```python
from build123d import *

# Parameters (mm, degrees)
F0_W     = 190
F0_H     = 10
F1_DEPTH = 20
F2_R     = 3
F2_W     = 150
F2_H     = 2
F3_DEPTH = 10
F4_R     = 2.5
F5_DEPTH = 10
F6_R     = 2.5
F7_DEPTH = 10


with BuildPart() as f1:
    # F0 (on Front) → F1 (new body)
    with BuildSketch(Plane.XZ):
        Rectangle(F0_W, F0_H)
    extrude(amount=F1_DEPTH)

    # F2 (on face) → F3 (cut)
    with BuildSketch(Plane.XY.offset(5)):
        with Locations((-56, -10)):
            Circle(F2_R)
        with Locations((-23.5, -10)):
            Circle(F2_R)
        with Locations((11.5, -10)):
            Circle(F2_R)
        with Locations((46, -10)):
            Circle(F2_R)
        with Locations((0, -19)):
            Rectangle(F2_W, F2_H)
    extrude(amount=-F3_DEPTH, mode=Mode.SUBTRACT)

    # F4 (on face) → F5 (cut)
    with BuildSketch(Plane(origin=(-95, 0, 0), x_dir=(0, -1, 0), z_dir=(-1, 0, 0))):
        with Locations((5, 0)):
            Circle(F4_R)
        with Locations((15, 0)):
            Circle(F4_R)
    extrude(amount=-F5_DEPTH, mode=Mode.SUBTRACT)

    # F6 (on face) → F7 (cut)
    with BuildSketch(Plane.YZ.offset(95)):
        with Locations((-5, 0)):
            Circle(F6_R)
        with Locations((-15, 0)):
            Circle(F6_R)
    extrude(amount=-F7_DEPTH, mode=Mode.SUBTRACT)


solid = f1.part
```
Check sheet for the modelled part. Datum: model origin and axes. Units: mm. A direction names the side the tool comes from. Round coordinates to 2 decimals unless told otherwise and drop trailing zeros. Order: outer loops, then holes, each group sorted by start corner. A loop starts at its lowest first (then second) coordinate and runs counter-clockwise, first axis right, second up. Notation, with made-up numbers: (30, 78) - (79, 78) arc R25 cw to (79, 92) - close; hole circle Ø1 at (-27, 21). An arc over 180 degrees is marked (long way). Answer as CSV lines item,"result". Start each with the question number.
1) Depth check by flat-ended pin: pin 1 (1.5 mm diameter, centred on y = -6, z = 0, fed in from +X); pin 2 (4 mm diameter, centred on x = 38.5, z = 2, fed in from -Y); pin 3 (1.5 mm diameter, centred on y = -5, z = 0.5, fed in from -X). Enter the tip coordinate at first touch or a pass-through.
2) Draft check along X on faces 1 (the face through (-1, 0, 0)), 2 (the face through (85, -5, 0)), 3 (the face through (-59, -10, 0)). Enter one of: +X half, -X half, draft (parallel to the pull), parting line (faces both ways), or undercut.
3) Scan lines: probe 1 along Y at (x, z) = (11.5, 2.5); probe 2 along X at (y, z) = (-11, 1.5); probe 3 along Z at (x, y) = (92.25, -15). Record each from-to range of solid material in increasing order.
4) Section check B-B (y = -5). Record the cut outline in (x, z).
5) Section check A-A (x = -23.5). Record the cut outline in (y, z), then the cut area to 3 significant figures.
6) Tool access check on faces 4 (the face through (90.1, -17.5, 0.1)), 5 (the face through (-1, -18, 0)), 6 (the face through (-90.1, -12.5, 0.1)), 7 (the face through (-85, -20, 0)). Record the directions out of +Z, -Z, +X, -X, +Y, -Y that give a thin tool (end or side, any length) a straight path to the whole face; none if there is none.
Determined:
1,pin 1,"x = 85"
1,pin 2,"y = -18"
1,pin 3,"x = -85"
2,face 1,"draft"
2,face 2,"+X half"
2,face 3,"undercut"
3,probe 1,"-18 to -13, -7 to 0"
3,probe 2,"-95 to -58.83, -53.17 to -26.33, -20.67 to 8.67, 14.33 to 43.17, 48.83 to 95"
3,probe 3,"-5 to -2.5, 2.5 to 5"
4,outline,"(-95, -5) - (95, -5) - (95, -2.5) - (85, -2.5) - (85, 2.5) - (95, 2.5) - (95, 5) - (-95, 5) - (-95, 2.5) - (-85, 2.5) - (-85, -2.5) - (-95, -2.5) - close"
5,outline,"(-18, -5) - (-13, -5) - (-13, 5) - (-18, 5) - close; (-7, -5) - (0, -5) - (0, 5) - (-7, 5) - close"
5,area,"120 mm^2"
6,face 4,"+X"
6,face 5,"+Z, -Z, -Y"
6,face 6,"-X"
6,face 7,"+Z, -Z, +X, -X, -Y"
